```python
from build123d import *

# Parameters (mm, degrees)
SKETCH1_W                = 32
SKETCH1_H                = 50
SKETCH1_R                = 5.5
SKETCH1_R_2              = 1.25
BOSS_EXTRUDE1_DEPTH      = 3.5
FILETE1_R                = 4
ESBO_O1_R                = 8
ESBO_O1_R_2              = 5.5
ESBO_O1_W                = 5.8
ESBO_O1_H                = 31.201183342
RESSALTO_EXTRUS_O1_DEPTH = 3
ESBO_O3_W                = 16.288942458
ESBO_O3_H                = 10.757575704
CORTE_EXTRUS_O1_DEPTH    = 30.887288268
CORTE_EXTRUS_O2_REACH    = 32.385
ESBO_O4_R                = 1.25
FILETE2_R                = 2


with BuildPart() as part:
    # Sketch1 → Boss-Extrude1 (new body)
    with BuildSketch(Plane(origin=(0, 0, 0), x_dir=(1, 0, 0), z_dir=(0, 1, 0))):
        Rectangle(SKETCH1_W, SKETCH1_H)
        with Locations(Location((0, 13.5, 0), (0, 0, 270))):
            Circle(SKETCH1_R, mode=Mode.SUBTRACT)
        with Locations(Location((13.5, 6.75, 0), (0, 0, 270))):
            Circle(SKETCH1_R_2, mode=Mode.SUBTRACT)
        with Locations(Location((13.5, -1.25, 0), (0, 0, 270))):
            Circle(SKETCH1_R_2, mode=Mode.SUBTRACT)
        with Locations(Location((13.5, -9.25, 0), (0, 0, 270))):
            Circle(SKETCH1_R_2, mode=Mode.SUBTRACT)
        with Locations(Location((13.5, -17.25, 0), (0, 0, 270))):
            Circle(SKETCH1_R_2, mode=Mode.SUBTRACT)
        with Locations(Location((-13.5, -17.25, 0), (0, 0, 90))):
            Circle(SKETCH1_R_2, mode=Mode.SUBTRACT)
        with Locations(Location((-13.5, -9.25, 0), (0, 0, 90))):
            Circle(SKETCH1_R_2, mode=Mode.SUBTRACT)
        with Locations(Location((-13.5, -1.25, 0), (0, 0, 90))):
            Circle(SKETCH1_R_2, mode=Mode.SUBTRACT)
        with Locations(Location((-13.5, 6.75, 0), (0, 0, 90))):
            Circle(SKETCH1_R_2, mode=Mode.SUBTRACT)
        Polygon((3.8, -15.5), (3.8, -11.8), (10.2, -11.8), (10.2, -19.2), (3.8, -19.2), align=None, mode=Mode.SUBTRACT)
        Polygon((-10.2, -19.2), (-3.8, -19.2), (-3.8, -15.5), (-3.8, -11.8), (-10.2, -11.8), align=None, mode=Mode.SUBTRACT)
    extrude(amount=BOSS_EXTRUDE1_DEPTH)

    # Filete1
    filete1_edges = [part.edges().sort_by_distance(p)[0] for p in [
        (16, 1.75, 25),
        (-16, 1.75, 25),
        (-16, 1.75, -25),
        (16, 1.75, -25),
    ]]
    fillet(filete1_edges, radius=FILETE1_R)

    # Esboço1 → Ressalto-extrusão1 (add)
    # profile 1 of 3: a face of its own
    with BuildSketch(Plane(origin=(0, 3.5, 0), x_dir=(1, 0, 0), z_dir=(0, 1, 0))):
        with Locations(Location((0, 13.5, 0), (0, 0, 90))):
            Circle(ESBO_O1_R)
        with Locations(Location((0, 13.5, 0), (0, 0, 270))):
            Circle(ESBO_O1_R_2, mode=Mode.SUBTRACT)
    # profile 2 of 3: a face of its own
    with BuildSketch(Plane(origin=(0, 3.5, 0), x_dir=(1, 0, 0), z_dir=(0, 1, 0))):
        with Locations((-13.1, -5.264208671)):
            Rectangle(ESBO_O1_W, ESBO_O1_H)
    # profile 3 of 3: a face of its own
    with BuildSketch(Plane(origin=(0, 3.5, 0), x_dir=(1, 0, 0), z_dir=(0, 1, 0))):
        with Locations((13.1, -5.264208671)):
            Rectangle(ESBO_O1_W, ESBO_O1_H)
    extrude(amount=RESSALTO_EXTRUS_O1_DEPTH)

    # Esboço3 → Corte-extrusão1 (cut, through all)
    with BuildSketch(Plane(origin=(0, 3.5, 0), x_dir=(1, 0, 0), z_dir=(0, 1, 0))):
        with Locations((0, -3.421212148)):
            Rectangle(ESBO_O3_W, ESBO_O3_H)
    extrude(amount=-CORTE_EXTRUS_O1_DEPTH, mode=Mode.SUBTRACT)

    # Esboço4 → Corte-extrusão2 (cut, up to next)
    with BuildSketch(Plane.XZ, mode=Mode.PRIVATE) as corte_extrus_o2_sk1:
        with Locations(Location((-13.5, 17.25, 0), (0, 0, 270))):
            Circle(ESBO_O4_R)
    corte_extrus_o2_tool1 = extrude(corte_extrus_o2_sk1.sketch, amount=-CORTE_EXTRUS_O2_REACH, mode=Mode.PRIVATE) & part.part
    # Esboço4 → Corte-extrusão2 (cut, up to next)
    with BuildSketch(Plane.XZ, mode=Mode.PRIVATE) as corte_extrus_o2_sk2:
        with Locations(Location((-13.5, 9.25, 0), (0, 0, 270))):
            Circle(ESBO_O4_R)
    corte_extrus_o2_tool2 = extrude(corte_extrus_o2_sk2.sketch, amount=-CORTE_EXTRUS_O2_REACH, mode=Mode.PRIVATE) & part.part
    # Esboço4 → Corte-extrusão2 (cut, up to next)
    with BuildSketch(Plane.XZ, mode=Mode.PRIVATE) as corte_extrus_o2_sk3:
        with Locations(Location((-13.5, 1.25, 0), (0, 0, 270))):
            Circle(ESBO_O4_R)
    corte_extrus_o2_tool3 = extrude(corte_extrus_o2_sk3.sketch, amount=-CORTE_EXTRUS_O2_REACH, mode=Mode.PRIVATE) & part.part
    # Esboço4 → Corte-extrusão2 (cut, up to next)
    with BuildSketch(Plane.XZ, mode=Mode.PRIVATE) as corte_extrus_o2_sk4:
        with Locations(Location((-13.5, -6.75, 0), (0, 0, 270))):
            Circle(ESBO_O4_R)
    corte_extrus_o2_tool4 = extrude(corte_extrus_o2_sk4.sketch, amount=-CORTE_EXTRUS_O2_REACH, mode=Mode.PRIVATE) & part.part
    # Esboço4 → Corte-extrusão2 (cut, up to next)
    with BuildSketch(Plane.XZ, mode=Mode.PRIVATE) as corte_extrus_o2_sk5:
        with Locations(Location((13.5, 1.25, 0), (0, 0, 270))):
            Circle(ESBO_O4_R)
    corte_extrus_o2_tool5 = extrude(corte_extrus_o2_sk5.sketch, amount=-CORTE_EXTRUS_O2_REACH, mode=Mode.PRIVATE) & part.part
    # Esboço4 → Corte-extrusão2 (cut, up to next)
    with BuildSketch(Plane.XZ, mode=Mode.PRIVATE) as corte_extrus_o2_sk6:
        with Locations(Location((13.5, 9.25, 0), (0, 0, 270))):
            Circle(ESBO_O4_R)
    corte_extrus_o2_tool6 = extrude(corte_extrus_o2_sk6.sketch, amount=-CORTE_EXTRUS_O2_REACH, mode=Mode.PRIVATE) & part.part
    # Esboço4 → Corte-extrusão2 (cut, up to next)
    with BuildSketch(Plane.XZ, mode=Mode.PRIVATE) as corte_extrus_o2_sk7:
        with Locations(Location((13.5, 17.25, 0), (0, 0, 270))):
            Circle(ESBO_O4_R)
    corte_extrus_o2_tool7 = extrude(corte_extrus_o2_sk7.sketch, amount=-CORTE_EXTRUS_O2_REACH, mode=Mode.PRIVATE) & part.part
    # Esboço4 → Corte-extrusão2 (cut, up to next)
    with BuildSketch(Plane.XZ, mode=Mode.PRIVATE) as corte_extrus_o2_sk8:
        with Locations(Location((13.5, -6.75, 0), (0, 0, 270))):
            Circle(ESBO_O4_R)
    corte_extrus_o2_tool8 = extrude(corte_extrus_o2_sk8.sketch, amount=-CORTE_EXTRUS_O2_REACH, mode=Mode.PRIVATE) & part.part
    add(corte_extrus_o2_tool1.solids().sort_by_distance((-13.5, 0, 17.25))[0], mode=Mode.SUBTRACT)
    add(corte_extrus_o2_tool2.solids().sort_by_distance((-13.5, 0, 9.25))[0], mode=Mode.SUBTRACT)
    add(corte_extrus_o2_tool3.solids().sort_by_distance((-13.5, 0, 1.25))[0], mode=Mode.SUBTRACT)
    add(corte_extrus_o2_tool4.solids().sort_by_distance((-13.5, 0, -6.75))[0], mode=Mode.SUBTRACT)
    add(corte_extrus_o2_tool5.solids().sort_by_distance((13.5, 0, 1.25))[0], mode=Mode.SUBTRACT)
    add(corte_extrus_o2_tool6.solids().sort_by_distance((13.5, 0, 9.25))[0], mode=Mode.SUBTRACT)
    add(corte_extrus_o2_tool7.solids().sort_by_distance((13.5, 0, 17.25))[0], mode=Mode.SUBTRACT)
    add(corte_extrus_o2_tool8.solids().sort_by_distance((13.5, 0, -6.75))[0], mode=Mode.SUBTRACT)

    # Filete2
    filete2_edges = [part.edges().sort_by_distance(p)[0] for p in [
        (-13.1, 3.5, 20.864800342),
        (-13.1, 3.5, -10.336383),
        (13.1, 3.5, -10.336383),
        (13.1, 3.5, 20.864800342),
        (0, 3.5, -5.5),
    ]]
    fillet(filete2_edges, radius=FILETE2_R)


solid = part.part
```
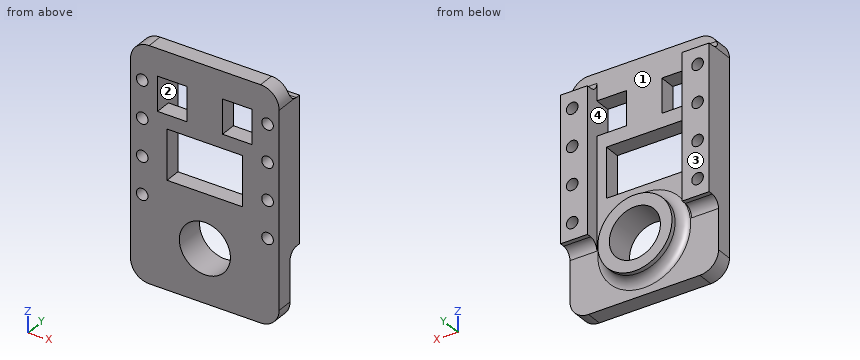
Geometry check sheet. Reference: the model listing, model coordinates, mm. Face numbers are marked on the shaded views. A direction names the side the tool comes from. Coordinates: 2 decimals unless noted, no trailing zeros. Loops run counter-clockwise (first coordinate to the right, second up) from the corner with the lowest first, then second, coordinate; pieces in that order, holes last. Notation, with made-up numbers: (34.5, 80.5) -> (76.5, 80.5) arc R11 ccw to (76.5, 94.5) -> close; hole circle Ø6 at (55, 38.25). An arc over 180 degrees is marked (long way). Put each result on its own line as item: value.
1) Thickness scan on line 1 (X direction, y = 2, z = 12); line 2 (X direction, y = 5.5, z = 9.25); line 3 (Z direction, x = 9.5, y = 1). Record the ranges inside material, lowest first.
Result set:
line 1: x = -16 to -10.2, -3.8 to 3.8, 10.2 to 16
line 2: x = -16 to -14.75, -12.25 to -10.2, 10.2 to 12.25, 14.75 to 16
line 3: z = -25 to 11.8, 19.2 to 25
2) Cross-section at C-C on x = 0. Record the boundary of the cut face in (y, z), plus the area to 3 significant figures.
Result set:
outline: (0, -25) -> (3.5, -25) -> (3.5, -23.5) arc R2 cw to (5.5, -21.5) -> (6.5, -21.5) -> (6.5, -19) -> (0, -19) -> close; (0, -8) -> (6.5, -8) -> (6.5, -5.5) -> (5.5, -5.5) arc R2 cw to (3.5, -3.5) -> (3.5, -1.96) -> (0, -1.96) -> close; (0, 8.8) -> (3.5, 8.8) -> (3.5, 25) -> (0, 25) -> close
area: 116 mm^2
3) Cross-section at D-D on y = 1.5. Count the separate pieces of the cut face and the enclosed holes in it, plus the area to 3 significant figures.
Result set:
separate pieces: 1
enclosed holes: 12
area: 1,180 mm^2
4) Gauge pin test, flat ends, axial feed: pin 1 Ø2 at (x, z) = (13.5, 1.25) entering from +Y; pin 2 Ø4 at (x, z) = (-13.5, -6.75) entering from -Y; pin 3 Ø0.8 at (x, y) = (14, 6) entering from +Z. Record the tip position at first contact, or that the pin passes through.
Result set:
pin 1: passes through
pin 2: stops at y = 0
pin 3: stops at z = 20.86
5) Cross-section at A-A on z = 17.25. Record the boundary of the cut face in (x, y), plus the area to 3 significant figures.
Result set:
outline: (-16, 0) -> (-14.75, 0) -> (-14.75, 6.5) -> (-16, 6.5) -> close; (-12.25, 0) -> (-10.2, 0) -> (-10.2, 6.5) -> (-12.25, 6.5) -> close; (-3.8, 0) -> (3.8, 0) -> (3.8, 3.5) -> (-3.8, 3.5) -> close; (10.2, 0) -> (12.25, 0) -> (12.25, 6.5) -> (10.2, 6.5) -> close; (14.75, 0) -> (16, 0) -> (16, 6.5) -> (14.75, 6.5) -> close
area: 69.5 mm^2
6) Cross-section at B-B on z = 1.25. Record the boundary of the cut face in (x, y).
Result set:
outline: (-16, 0) -> (-14.75, 0) -> (-14.75, 6.5) -> (-16, 6.5) -> close; (-12.25, 0) -> (-8.14, 0) -> (-8.14, 3.5) -> (-10.2, 3.5) -> (-10.2, 6.5) -> (-12.25, 6.5) -> close; (8.14, 0) -> (12.25, 0) -> (12.25, 6.5) -> (10.2, 6.5) -> (10.2, 3.5) -> (8.14, 3.5) -> close; (14.75, 0) -> (16, 0) -> (16, 6.5) -> (14.75, 6.5) -> close
7) Tool access check on the marked faces 3 and 4. Record the directions out of +Z, -Z, +X, -X, +Y, -Y that give a thin tool (end or side, any length) a straight path to the whole face; none if there is none.
Result set:
face 3: +Z, -Z, +X, -X, +Y
face 4: +Y
8) Release check for a two-part mould opening along Z. For the marked faces 1 and 2 record: released by +Z, released by -Z, zero draft, split by the parting line, or undercut.
Result set:
face 1: zero draft
face 2: undercut
